```python
from build123d import *

# Parameters (mm, degrees)
BOSS_EXTRUDE2_REACH             = 105.962
BOSS_EXTRUDE2_END_RADIUS        = 179.3875
SKETCH2_R                       = 4.191
SKETCH2_R_2                     = 3.175
BOSS_EXTRUDE2_DIRECTION_2_DEPTH = 22.86
SKETCH2_6_R                     = 72.587717307
SKETCH2_6_R_2                   = 41.148
SKETCH2_6_R_3                   = 12.7
CUT_EXTRUDE3_DEPTH              = 106.169068821
CUT_EXTRUDE4_DEPTH              = 63.521159814
CUT_EXTRUDE4_DEPTH_BACK         = 63.521159814
SKETCH2_8_R                     = 3.175


with BuildPart() as part:
    # Sketch1 → Revolve1 (revolve)
    with BuildSketch(Plane.XY, mode=Mode.PRIVATE) as revolve1_sk:
        with BuildLine():
            Line((0, 1.5875), (0, 0))
            ThreePointArc((0, 0), (-37.095674447, 3.877425948), (-72.587717307, 15.342084177))
            Line((-72.587717307, 15.342084177), (-71.138583931, 16.439220241))
            ThreePointArc((-71.138583931, 16.439220241), (-36.336179346, 5.340029261), (0, 1.5875))
        make_face()
    revolve(revolve1_sk.sketch.rotate(Axis((0, 0, 0), (0, 1, 0)), 270), axis=Axis((0, 0, 0), (0, 1, 0)))

    # Boss-Extrude2: up to this sphere (the profile starts outside it)
    boss_extrude2_end = Location((0, 179.3875, 0)) * Sphere(BOSS_EXTRUDE2_END_RADIUS, mode=Mode.PRIVATE)
    # Sketch2 → Boss-Extrude2 (add, up to the surface)
    with BuildSketch(Plane(origin=(0, 0, 0), x_dir=(1, 0, 0), z_dir=(0, 1, 0)), mode=Mode.PRIVATE) as boss_extrude2_sk1:
        with Locations(Location((-28.575, 0, 0), (0, 0, 270))):
            Circle(SKETCH2_R)
        with Locations((-28.575, 0)):
            Circle(SKETCH2_R_2, mode=Mode.SUBTRACT)
    boss_extrude2_tool1 = extrude(boss_extrude2_sk1.sketch, amount=BOSS_EXTRUDE2_REACH, mode=Mode.PRIVATE) - boss_extrude2_end
    add(boss_extrude2_tool1.solids().sort_by_distance((-28.575, 0, -4.072461))[0])
    # Sketch2 → Boss-Extrude2 (add, up to the surface)
    with BuildSketch(Plane(origin=(0, 0, 0), x_dir=(1, 0, 0), z_dir=(0, 1, 0)), mode=Mode.PRIVATE) as boss_extrude2_sk2:
        with Locations((-28.575, 0)):
            Circle(SKETCH2_R_2)
    boss_extrude2_tool2 = extrude(boss_extrude2_sk2.sketch, amount=BOSS_EXTRUDE2_REACH, mode=Mode.PRIVATE) - boss_extrude2_end
    add(boss_extrude2_tool2.solids().sort_by_distance((-28.575, 0, 0))[0])
    # Sketch2 → Boss-Extrude2 (add, up to the surface)
    with BuildSketch(Plane(origin=(0, 0, 0), x_dir=(1, 0, 0), z_dir=(0, 1, 0)), mode=Mode.PRIVATE) as boss_extrude2_sk3:
        with Locations(Location((0, 28.575, 0), (0, 0, 270))):
            Circle(SKETCH2_R)
        with Locations((0, 28.575)):
            Circle(SKETCH2_R_2, mode=Mode.SUBTRACT)
    boss_extrude2_tool3 = extrude(boss_extrude2_sk3.sketch, amount=BOSS_EXTRUDE2_REACH, mode=Mode.PRIVATE) - boss_extrude2_end
    add(boss_extrude2_tool3.solids().sort_by_distance((0, 0, -32.647461))[0])
    # Sketch2 → Boss-Extrude2 (add, up to the surface)
    with BuildSketch(Plane(origin=(0, 0, 0), x_dir=(1, 0, 0), z_dir=(0, 1, 0)), mode=Mode.PRIVATE) as boss_extrude2_sk4:
        with Locations((0, 28.575)):
            Circle(SKETCH2_R_2)
    boss_extrude2_tool4 = extrude(boss_extrude2_sk4.sketch, amount=BOSS_EXTRUDE2_REACH, mode=Mode.PRIVATE) - boss_extrude2_end
    add(boss_extrude2_tool4.solids().sort_by_distance((0, 0, -28.575))[0])
    # Sketch2 → Boss-Extrude2 (add, up to the surface)
    with BuildSketch(Plane(origin=(0, 0, 0), x_dir=(1, 0, 0), z_dir=(0, 1, 0)), mode=Mode.PRIVATE) as boss_extrude2_sk5:
        with Locations(Location((28.575, 0, 0), (0, 0, 270))):
            Circle(SKETCH2_R)
        with Locations((28.575, 0)):
            Circle(SKETCH2_R_2, mode=Mode.SUBTRACT)
    boss_extrude2_tool5 = extrude(boss_extrude2_sk5.sketch, amount=BOSS_EXTRUDE2_REACH, mode=Mode.PRIVATE) - boss_extrude2_end
    add(boss_extrude2_tool5.solids().sort_by_distance((28.575, 0, -4.072461))[0])
    # Sketch2 → Boss-Extrude2 (add, up to the surface)
    with BuildSketch(Plane(origin=(0, 0, 0), x_dir=(1, 0, 0), z_dir=(0, 1, 0)), mode=Mode.PRIVATE) as boss_extrude2_sk6:
        with Locations((28.575, 0)):
            Circle(SKETCH2_R_2)
    boss_extrude2_tool6 = extrude(boss_extrude2_sk6.sketch, amount=BOSS_EXTRUDE2_REACH, mode=Mode.PRIVATE) - boss_extrude2_end
    add(boss_extrude2_tool6.solids().sort_by_distance((28.575, 0, 0))[0])
    # Sketch2 → Boss-Extrude2 (add, up to the surface)
    with BuildSketch(Plane(origin=(0, 0, 0), x_dir=(1, 0, 0), z_dir=(0, 1, 0)), mode=Mode.PRIVATE) as boss_extrude2_sk7:
        with Locations(Location((0, -28.575, 0), (0, 0, 270))):
            Circle(SKETCH2_R)
        with Locations((0, -28.575)):
            Circle(SKETCH2_R_2, mode=Mode.SUBTRACT)
    boss_extrude2_tool7 = extrude(boss_extrude2_sk7.sketch, amount=BOSS_EXTRUDE2_REACH, mode=Mode.PRIVATE) - boss_extrude2_end
    add(boss_extrude2_tool7.solids().sort_by_distance((0, 0, 24.502539))[0])
    # Sketch2 → Boss-Extrude2 (add, up to the surface)
    with BuildSketch(Plane(origin=(0, 0, 0), x_dir=(1, 0, 0), z_dir=(0, 1, 0)), mode=Mode.PRIVATE) as boss_extrude2_sk8:
        with Locations((0, -28.575)):
            Circle(SKETCH2_R_2)
    boss_extrude2_tool8 = extrude(boss_extrude2_sk8.sketch, amount=BOSS_EXTRUDE2_REACH, mode=Mode.PRIVATE) - boss_extrude2_end
    add(boss_extrude2_tool8.solids().sort_by_distance((0, 0, 28.575))[0])

    # Sketch2 → Boss-Extrude2 direction 2 (add)
    # profile 1 of 8: a face of its own
    with BuildSketch(Plane(origin=(0, 0, 0), x_dir=(1, 0, 0), z_dir=(0, 1, 0))):
        with Locations(Location((-28.575, 0, 0), (0, 0, 270))):
            Circle(SKETCH2_R)
        with Locations((-28.575, 0)):
            Circle(SKETCH2_R_2, mode=Mode.SUBTRACT)
    # profile 2 of 8: a face of its own
    with BuildSketch(Plane(origin=(0, 0, 0), x_dir=(1, 0, 0), z_dir=(0, 1, 0))):
        with Locations((-28.575, 0)):
            Circle(SKETCH2_R_2)
    # profile 3 of 8: a face of its own
    with BuildSketch(Plane(origin=(0, 0, 0), x_dir=(1, 0, 0), z_dir=(0, 1, 0))):
        with Locations(Location((0, 28.575, 0), (0, 0, 270))):
            Circle(SKETCH2_R)
        with Locations((0, 28.575)):
            Circle(SKETCH2_R_2, mode=Mode.SUBTRACT)
    # profile 4 of 8: a face of its own
    with BuildSketch(Plane(origin=(0, 0, 0), x_dir=(1, 0, 0), z_dir=(0, 1, 0))):
        with Locations((0, 28.575)):
            Circle(SKETCH2_R_2)
    # profile 5 of 8: a face of its own
    with BuildSketch(Plane(origin=(0, 0, 0), x_dir=(1, 0, 0), z_dir=(0, 1, 0))):
        with Locations(Location((28.575, 0, 0), (0, 0, 270))):
            Circle(SKETCH2_R)
        with Locations((28.575, 0)):
            Circle(SKETCH2_R_2, mode=Mode.SUBTRACT)
    # profile 6 of 8: a face of its own
    with BuildSketch(Plane(origin=(0, 0, 0), x_dir=(1, 0, 0), z_dir=(0, 1, 0))):
        with Locations((28.575, 0)):
            Circle(SKETCH2_R_2)
    # profile 7 of 8: a face of its own
    with BuildSketch(Plane(origin=(0, 0, 0), x_dir=(1, 0, 0), z_dir=(0, 1, 0))):
        with Locations(Location((0, -28.575, 0), (0, 0, 270))):
            Circle(SKETCH2_R)
        with Locations((0, -28.575)):
            Circle(SKETCH2_R_2, mode=Mode.SUBTRACT)
    # profile 8 of 8: a face of its own
    with BuildSketch(Plane(origin=(0, 0, 0), x_dir=(1, 0, 0), z_dir=(0, 1, 0))):
        with Locations((0, -28.575)):
            Circle(SKETCH2_R_2)
    extrude(amount=-BOSS_EXTRUDE2_DIRECTION_2_DEPTH)

    # Sketch2<6> → Cut-Extrude3 (cut, through all)
    # profile 1 of 2: a face of its own
    with BuildSketch(Plane(origin=(0, 0, 0), x_dir=(1, 0, 0), z_dir=(0, 1, 0))):
        Circle(SKETCH2_6_R)
        Circle(SKETCH2_6_R_2, mode=Mode.SUBTRACT)
    # profile 2 of 2: a face of its own
    with BuildSketch(Plane(origin=(0, 0, 0), x_dir=(1, 0, 0), z_dir=(0, 1, 0))):
        Circle(SKETCH2_6_R_3)
    extrude(amount=CUT_EXTRUDE3_DEPTH, mode=Mode.SUBTRACT)


with BuildPart() as cut_extrude3_kept_piece:
    # of the separate pieces the step leaves, the one the design keeps (cut_extrude3_pieces_kept)
    add(part.part.solids().sort_by_distance((41.148, 6.414432455, 0))[0])

    # Sketch2<8> → Cut-Extrude4 (cut, two sides: drawn at the far end of the back side and taken through both)
    with BuildSketch(Plane(origin=(0, 0, 0), x_dir=(1, 0, 0), z_dir=(0, 1, 0)).offset(-CUT_EXTRUDE4_DEPTH_BACK)):
        with Locations(Location((-28.575, 0, 0), (0, 0, 270))):
            Circle(SKETCH2_8_R)
        with Locations(Location((0, 28.575, 0), (0, 0, 270))):
            Circle(SKETCH2_8_R)
        with Locations(Location((28.575, 0, 0), (0, 0, 270))):
            Circle(SKETCH2_8_R)
        with Locations(Location((0, -28.575, 0), (0, 0, 270))):
            Circle(SKETCH2_8_R)
    extrude(amount=CUT_EXTRUDE4_DEPTH + CUT_EXTRUDE4_DEPTH_BACK, mode=Mode.SUBTRACT)


solid = cut_extrude3_kept_piece.part
```
Model file for the job. Use its own axes, mm. Coordinates: 2 decimals unless noted, no trailing zeros. Loops run counter-clockwise (first coordinate to the right, second up) from the corner with the lowest first, then second, coordinate; pieces in that order, holes last. Notation, with made-up numbers: (-1.75, 45.25) -> (35.25, 45.25) arc R20 ccw to (35.25, 59.25) -> close; hole circle Ø6 at (-6.75, 49). An arc over 180 degrees is marked (long way). Answer as a JSON object with one key per item and string values.
Q1. Cut at B-B (z = 8). List the corners of the cut face in (x, y), and give its area (3 significant figures).
Report:
{"outline": "(-40.36, 4.78) arc R179.21 ccw to (-9.86, 0.45) -> (-9.86, 2.04) arc R177.62 cw to (-40.36, 6.41) -> close; (9.86, 0.45) arc R179.21 ccw to (40.36, 4.78) -> (40.36, 6.41) arc R177.62 cw to (9.86, 2.04) -> close", "area": "98.0 mm2"}
Q2. Flat gauge pins, fed straight in: P1, Ø7.5, axis at x = 28.575, z = 0, coming from the +Y side; P2, Ø3, axis at x = 21, z = 31.5, coming from the +Y side; P3, Ø8.5, axis at x = -28.575, z = 0, coming from the -Y side; P4, Ø10, axis at x = -0.5, y = -17.5, coming from the +Z side. Where does each tip first touch, or does it go through?
Report:
{"P1": "stops at y = 4.55", "P2": "stops at y = 6", "P3": "stops at y = -22.86", "P4": "stops at z = 32.77"}
Q3. Probe probe 1 along Z at (x, y) = (-0.5, -2.5); probe 2 along Z at (x, y) = (2, -6.5); probe 3 along Z at (x, y) = (28, -17.75). List the from-to ranges inside material, lowest first.
Report:
{"probe 1": "z = -32.74 to -31.71, -25.44 to -24.41, 24.41 to 25.44, 31.71 to 32.74", "probe 2": "z = -32.26 to -31.04, -26.11 to -24.89, 24.89 to 26.11, 31.04 to 32.26", "probe 3": "z = -4.15 to -3.12, 3.12 to 4.15"}
Q4. Cut at D-D (z = -22). List the corners of the cut face in (x, y), and give its area (3 significant figures).
Report:
{"outline": "(-34.77, 4.78) arc R178.03 ccw to (34.77, 4.78) -> (34.77, 6.41) arc R176.43 cw to (-34.77, 6.41) -> close", "area": "112 mm2"}
Q5. Cut at A-A (y = -4.5). List the corners of the cut face in (x, z) (3 decimals), and give its area (3 significant figures).
Report:
{"outline": "circle Ø8.382 at (-28.575, 0); circle Ø8.382 at (0, -28.575); circle Ø8.382 at (0, 28.575); circle Ø8.382 at (28.575, 0); hole circle Ø6.35 at (-28.575, 0); hole circle Ø6.35 at (0, -28.575); hole circle Ø6.35 at (0, 28.575); hole circle Ø6.35 at (28.575, 0)", "area": "94.0 mm2"}
Q6. Pull direction Y, two halves, no side cores. Call faces 1 (the flat face through (1, -22.86, 25)), 2 (the cylindrical face through (2.146, -9.398, -30.915)): released by +Y, released by -Y, zero draft, split by the parting line, or undercut.
Report:
{"face 1": "released by -Y", "face 2": "zero draft"}
Q7. Cut at C-C (x = 0). State how many separate pieces and enclosed holes the cut face has, and give its area (3 significant figures).
Report:
{"separate pieces": "4", "enclosed holes": "0", "area": "173 mm2"}
